Check sheet for the modelled part. Datum: model origin and axes. Units: mm. Face numbers are marked on the shaded views. Give positions to 0.01 mm unless a question says otherwise; leave off trailing zeros. Write each loop counter-clockwise with the first axis right and the second up, starting at its lowest first coordinate (ties: lowest second). Pieces come first, ordered by that corner, then holes.
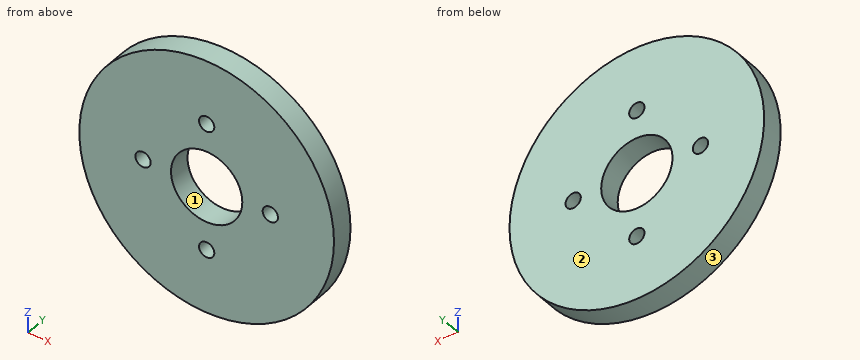
from build123d import *

# Parameters (mm, degrees)
F0_R     = 100
F0_R_2   = 28
F1_DEPTH = 18
F2_D     = 12


with BuildPart() as f1:
    # F0 (on Front) → F1 (new body)
    with BuildSketch(Plane.XZ):
        Circle(F0_R)
        Circle(F0_R_2, mode=Mode.SUBTRACT)
    extrude(amount=F1_DEPTH)

    # F2 (through all)
    with Locations(Plane(origin=(0, 0, 0), x_dir=(1, 0, 0), z_dir=(0, 1, 0))):
        with Locations((0, 50), (50, 0), (0, -50), (-50, 0)):
            Hole(F2_D / 2)


solid = f1.part
1) Sectioned sample at A-A on z = 0. Record the boundary of the cut face in (x, y).
2) Scan lines: L1, parallel to Z at x = 1.5, y = -3.5; L2, parallel to Z at x = 47, y = -13.25; L3, parallel to Z at x = 6.5, y = -17. Record each from-to range of solid material in increasing order.
3) Gauge pin test, flat ends, axial feed: pin 1 (5 mm diameter, centred on y = -2.5, z = 65.5, fed in from +X); pin 2 (8 mm diameter, centred on x = 16, y = -13.5, fed in from -Z); pin 3 (4 mm diameter, centred on x = -60.5, y = -7.5, fed in from +Z); pin 4 (11 mm diameter, centred on x = 0, z = -50, fed in from +Y). Record the tip position at first contact, or that the pin passes through.
4) Sectioned sample at B-B on y = -11.25. Record the boundary of the cut face in (x, z).
5) Sectioned sample at D-D on z = 50. Record the boundary of the cut face in (x, y).
6) Draft check along Z on the marked faces 1, 2 and 3. Enter one of: +Z half, -Z half, draft (parallel to the pull), parting line (faces both ways), or undercut.
7) Sectioned sample at C-C on x = 17.5. Record the boundary of the cut face in (y, z).
Answers below:
1. outline: (-100, -18) - (-56, -18) - (-56, 0) - (-100, 0) - close; (-44, -18) - (-28, -18) - (-28, 0) - (-44, 0) - close; (28, -18) - (44, -18) - (44, 0) - (28, 0) - close; (56, -18) - (100, -18) - (100, 0) - (56, 0) - close
2. L1: z = -99.99 to -55.81, -44.19 to -27.96, 27.96 to 44.19, 55.81 to 99.99
2. L2: z = -88.27 to -5.2, 5.2 to 88.27
2. L3: z = -99.79 to -27.24, 27.24 to 99.79
3. pin 1: stops at x = 77.66
3. pin 2: stops at z = -99.28
3. pin 3: stops at z = 81.1
3. pin 4: passes through
4. outline: circle Ø200 at (0, 0); hole circle Ø12 at (-50, 0); hole circle Ø56 at (0, 0); hole circle Ø12 at (0, -50); hole circle Ø12 at (0, 50); hole circle Ø12 at (50, 0)
5. outline: (-86.6, -18) - (-6, -18) - (-6, 0) - (-86.6, 0) - close; (6, -18) - (86.6, -18) - (86.6, 0) - (6, 0) - close
6. face 1: undercut
6. face 2: draft
6. face 3: parting line
7. outline: (-18, -98.46) - (0, -98.46) - (0, -21.86) - (-18, -21.86) - close; (-18, 21.86) - (0, 21.86) - (0, 98.46) - (-18, 98.46) - close
